Here's how the part is built. I have some questions about the finished solid (model axes, mm). A direction names the side the tool comes from. Round coordinates to 2 decimals unless told otherwise and drop trailing zeros. Order: outer loops, then holes, each group sorted by start corner. A loop starts at its lowest first (then second) coordinate and runs counter-clockwise, first axis right, second up. Notation, with made-up numbers: (51, 66) -> (94, 66) arc R19 ccw to (94, 102) -> close; hole circle Ø10 at (31, 83.25). An arc over 180 degrees is marked (long way). One line per item, written item: value.
```python
from build123d import *

# Parameters (mm, degrees)
F1_DEPTH = 84.0288382024
F4_W     = 52.5419712067
F4_H     = 82.2811126709


with BuildPart() as f1:
    # F0 (on Front) → F1 (new body)
    with BuildSketch(Plane.XZ):
        Polygon((58.445379138, -63.900783658), (-53.5063222051, 52.4989590049), (-53.5063222051, -63.900783658), align=None)
    extrude(amount=F1_DEPTH)

    # F4 (on offset) → F5 (join, up to the next surface of F1)
    with BuildSketch(Plane.YZ.offset(134.6250604838)):
        with Locations((-39.9457663298, -12.7352923155)):
            Rectangle(F4_W, F4_H)
    extrude(until=Until.NEXT, dir=(-1, 0, 0))


solid = f1.part
```
Q1. I want a section at B-B on x = 11. Write out the boundary of the cut face in (y, z).
Answers:
outline: (-84.03, -63.9) -> (0, -63.9) -> (0, -14.57) -> (-13.67, -14.57) -> (-13.67, 28.41) -> (-66.22, 28.41) -> (-66.22, -14.57) -> (-84.03, -14.57) -> close
Q2. I want a section at A-A on y = -33.5. Write out the boundary of the cut face in (x, z).
Answers:
outline: (-53.51, -63.9) -> (58.45, -63.9) -> (48.8, -53.88) -> (134.63, -53.88) -> (134.63, 28.41) -> (-30.33, 28.41) -> (-53.51, 52.5) -> close
Q3. For P1, Ø2, axis at x = 106.5, y = -31.5, coming from the -Z side; P2, Ø24.5, axis at x = 24, z = 6.5, coming from the +Y side; P3, Ø3, axis at x = -11, y = -74, coming from the +Z side, each with a flat end and sliding along its axis, tell me the tip position at first contact or that it passes through.
Answers:
P1: z = -53.88
P2: y = -13.67
P3: z = 9.86
Q4. I need wall thicknesses on line 1 along Z through (x, y) = (68.5, -63.5); line 2 along Y through (x, z) = (109.5, -49.5); line 3 along Z through (x, y) = (35.5, -20). Which ranges of each line are inside material? Lowest first, please.
Answers:
line 1: -53.88 to 28.41
line 2: -66.22 to -13.67
line 3: -63.9 to 28.41
Q5. Which directions (+Z, -Z, +X, -X, +Y, -Y) give clear straight access to the entire face, cutting with the end or side of a thin tool? Please do faces 1 (the face through (72, -13.675, -13)), 2 (the face through (-53.506, -41, -5)), 3 (the face through (72, -66.217, -13)), 4 (the face through (53, -40, 28.405)), 5 (the face through (134.625, -40, -12)).
Answers:
face 1: +Z, +X, +Y
face 2: +Z, -Z, -X, +Y, -Y
face 3: +Z, +X, -Y
face 4: +Z, +X, +Y, -Y
face 5: +Z, -Z, +X, +Y, -Y
Q6. I want a section at C-C on z = 15.5. Write out the boundary of the cut face in (x, y), then the cut area to 3 significant figures.
Answers:
outline: (-53.51, -84.03) -> (-17.92, -84.03) -> (-17.92, -66.22) -> (134.63, -66.22) -> (134.63, -13.67) -> (-17.92, -13.67) -> (-17.92, 0) -> (-53.51, 0) -> close
area: 11,000 mm2
Q7. I want a section at D-D on x = 78. Write out the boundary of the cut face in (y, z), then the cut area to 3 significant figures.
Answers:
outline: (-66.22, -53.88) -> (-13.67, -53.88) -> (-13.67, 28.41) -> (-66.22, 28.41) -> close
area: 4,320 mm2
